```python
from build123d import *

# Parameters (mm, degrees)
F0_W     = 584.2
F0_H     = 152.4
F1_DEPTH = 3.175
F2_R     = 63.5
F3_DEPTH = 25.4
F4_R     = 65.0875
F4_R_2   = 63.5
F5_DEPTH = 127


with BuildPart() as f1:
    # F0 (on Right) → F1 (new body)
    with BuildSketch(Plane.YZ):
        Rectangle(F0_W, F0_H)
    extrude(amount=F1_DEPTH)

    # F2 (on face) → F3 (cut)
    with BuildSketch(Plane.YZ.offset(3.175)):
        with Locations((165.1, 0)):
            Circle(F2_R)
    extrude(amount=-F3_DEPTH, mode=Mode.SUBTRACT)

    # F4 (on face) → F5 (join)
    with BuildSketch(Plane.YZ.offset(3.175)):
        with Locations((165.1, 0)):
            Circle(F4_R)
        with Locations((165.1, 0)):
            Circle(F4_R_2, mode=Mode.SUBTRACT)
    extrude(amount=F5_DEPTH)


solid = f1.part
```
CAD build for the part. Positions are in the model's coordinates, mm. A direction names the side the tool comes from. Coordinates: 2 decimals unless noted, no trailing zeros. Order: outer loops, then holes, each group sorted by start corner. A loop starts at its lowest first (then second) coordinate and runs counter-clockwise, first axis right, second up. Notation, with made-up numbers: (22.5, -12.75) - (32.5, -12.75) arc R20 cw to (32.5, 7.25) - close; hole circle Ø5 at (37.25, -34.75). An arc over 180 degrees is marked (long way). Use a Markdown table: item, result. Add a question column.
(1) Saw through at B-B (y = 165.1). Give the cut face in (x, z) (1 decimal).
(2) Saw through at C-C (x = 56). Give the cut face in (y, z) (1 decimal).
(3) Which spindle directions (+Z, -Z, +X, -X, +Y, -Y) get a long thin tool onto all of the face, cutting with end or side? Do faces 1 (the face through (130.175, 179.3, -62.4)), 2 (the face through (65.79, 227.18, 19.55)). Say none if no direction does.
(4) Flat gauge pins, fed straight in: pin 1 (1 mm diameter, centred on x = 113.5, z = -10.5, fed in from +Y); pin 2 (12 mm diameter, centred on y = 25, z = 35, fed in from +X) (3 decimals); pin 3 (3 mm diameter, centred on x = 41.5, y = 224, fed in from +Z). Where does each tip first touch, or does it go through?
(5) Saw through at A-A (z = 0). Give the cut face in (x, y) (1 decimal).
(6) Saw through at D-D (y = -178). Give the cut face in (x, z) (3 decimals), then the cut area to 3 significant figures.
(7) Drill centre lines: line 1 along Z through (x, y) = (2.05, 165.1); line 2 along Z through (x, y) = (77, 165.1); line 3 along X through (y, z) = (-22.5, 25.5) (3 decimals). Where is each one in solid material? Low to high. Write a range as [from, to].
Solved:
| question | item | result |
|---|---|---|
| 1 | outline | (0, -76.2) - (3.2, -76.2) - (3.2, -65.1) - (130.2, -65.1) - (130.2, -63.5) - (0, -63.5) - close; (0, 63.5) - (130.2, 63.5) - (130.2, 65.1) - (3.2, 65.1) - (3.2, 76.2) - (0, 76.2) - close |
| 2 | outline | circle Ø130.2 at (165.1, 0); hole circle Ø127 at (165.1, 0) |
| 3 | face 1 | +Z, -Z, +X, +Y, -Y |
| 3 | face 2 | +X |
| 4 | pin 1 | stops at y = 229.41 |
| 4 | pin 2 | stops at x = 3.175 |
| 4 | pin 3 | stops at z = 30.69 |
| 5 | outline | (0, -292.1) - (3.2, -292.1) - (3.2, 100) - (130.2, 100) - (130.2, 101.6) - (0, 101.6) - close; (0, 228.6) - (130.2, 228.6) - (130.2, 230.2) - (3.2, 230.2) - (3.2, 292.1) - (0, 292.1) - close |
| 6 | outline | (0, -76.2) - (3.175, -76.2) - (3.175, 76.2) - (0, 76.2) - close |
| 6 | area | 484 mm² |
| 7 | line 1 | z = [-76.2, -63.5], [63.5, 76.2] |
| 7 | line 2 | z = [-65.09, -63.5], [63.5, 65.09] |
| 7 | line 3 | x = [0, 3.175] |
